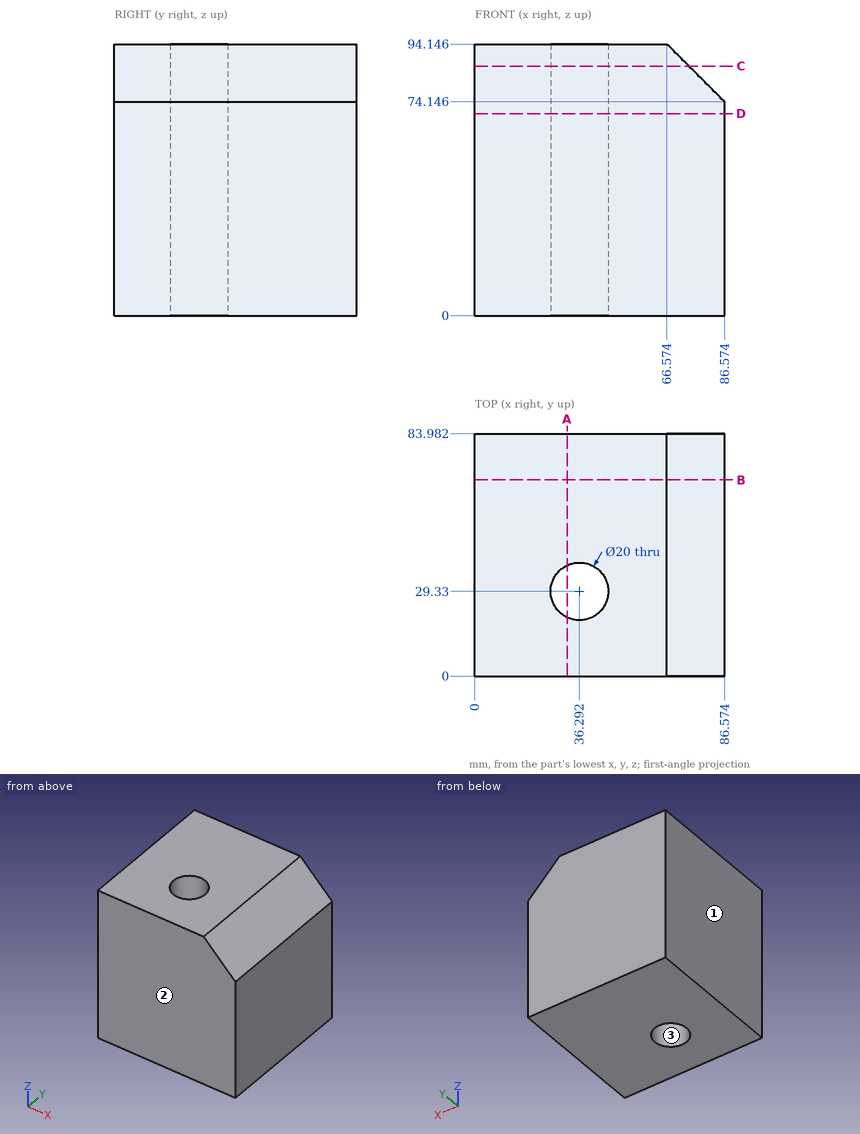
Check sheet for the drawn part. Datum: minimum x, y, z corner. Units: mm. Give positions to 0.01 mm unless a question says otherwise; leave off trailing zeros. Loops run counter-clockwise (first coordinate to the right, second up) from the corner with the lowest first, then second, coordinate; pieces in that order, holes last. Notation, with made-up numbers: M -19.5,-22 L 37.5,-22 A36 cw 37.5,17 Z; hole C -7,-24 d7. An arc over 180 degrees is marked long. Return JSON: item names as keys, results as strings.
1) Section check A-A, the plane x = 32. Enter the section's corners in (y, z), and give its area (3 significant figures).
Findings:
{"outline": "M 0,0 L 20.3,0 L 20.3,94.15 L 0,94.15 Z; M 38.36,0 L 83.98,0 L 83.98,94.15 L 38.36,94.15 Z", "area": "6,210 mm2"}
2) Section check B-B, the plane y = 68. Enter the section's corners in (x, z) (1 decimal).
Findings:
{"outline": "M 0,0 L 86.6,0 L 86.6,74.1 L 66.6,94.1 L 0,94.1 Z"}
3) Section check D-D, the plane z = 70. Enter the section's corners in (x, y) (1 decimal).
Findings:
{"outline": "M 0,0 L 86.6,0 L 86.6,84 L 0,84 Z; hole C 36.3,29.3 d20"}
4) Material ranges on L1, parallel to X at y = 29.5, z = 36.5 (1 decimal); L2, parallel to Y at x = 38, z = 25.5; L3, parallel to Y at x = 45, z = 62.5 (1 decimal), recorded low to high. Write a range as [from, to].
Findings:
{"L1": "x = [0, 26.3], [46.3, 86.6]", "L2": "y = [0, 19.48], [39.18, 83.98]", "L3": "y = [0, 24.4], [34.2, 84]"}
5) Mould release check, pull along Y, two halves, no side actions. Record for the marked faces 1, 2 and 3: released by +Y, released by -Y, zero draft, split by the parting line, or undercut.
Findings:
{"face 1": "zero draft", "face 2": "released by -Y", "face 3": "undercut"}
6) Section check C-C, the plane z = 86.5. Enter the section's corners in (x, y).
Findings:
{"outline": "M 0,0 L 74.22,0 L 74.22,83.98 L 0,83.98 Z; hole C 36.29,29.33 d20"}
